Verification items for this drawing (mm, ordinates from the low corner). A direction names the side the tool comes from. Round coordinates to 2 decimals unless told otherwise and drop trailing zeros. Write each loop counter-clockwise with the first axis right and the second up, starting at its lowest first coordinate (ties: lowest second). Pieces come first, ordered by that corner, then holes. Notation, with made-up numbers: (-25, 48) -> (21, 48) arc R20 ccw to (21, 87) -> close; hole circle Ø5 at (60.5, 65). An arc over 180 degrees is marked (long way). Put each result on its own line as item: value. Start each with the question number.
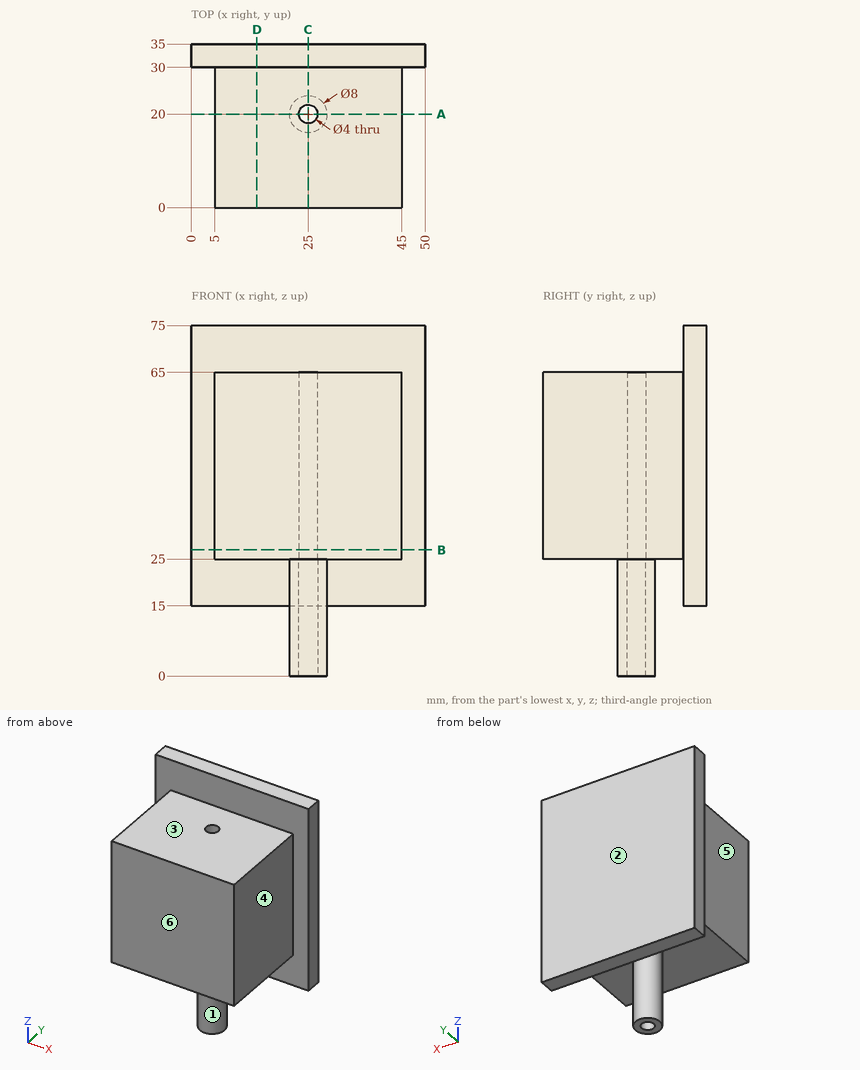
(1) Mould release check, pull along Y, two halves, no side actions. Record for the marked faces 1, 2 and 3: +Y half, -Y half, draft (parallel to the pull), parting line (faces both ways), or undercut.
(2) Sectioned sample at A-A (y = 20). Record the cut outline in (x, z).
(3) Go/stop test with flat-tipped pins: pin 1 Ø1.5 at (x, z) = (29, 10.5) entering from -Y; pin 2 Ø5.5 at (x, y) = (21, 32) entering from -Z; pin 3 Ø3 at (y, z) = (16, 16) entering from +X. Record where each tip stops, or that it passes through.
(4) Sectioned sample at D-D (x = 14). Record the cut outline in (y, z).
(5) Sectioned sample at C-C (x = 25). Record the cut outline in (y, z), and give its area (3 significant figures).
(6) Material ranges on L1, parallel to Y at x = 25, z = 52; L2, parallel to Y at x = 25, z = 6.5; L3, parallel to X at y = 20, z = 34, recorded low to high. Write a range as from..to.
(7) Set-up check for the marked faces 4, 5 and 6: record each of +Z, -Z, +X, -X, +Y, -Y from which the full face is reachable in a straight line by a thin tool's end or side.
(8) Sectioned sample at B-B (z = 27). Record the cut outline in (x, y).
Found:
1. face 1: undercut
1. face 2: +Y half
1. face 3: draft
2. outline: (5, 25) -> (21, 25) -> (21, 0) -> (23, 0) -> (23, 65) -> (5, 65) -> close; (27, 0) -> (29, 0) -> (29, 25) -> (45, 25) -> (45, 65) -> (27, 65) -> close
3. pin 1: y = 17.67
3. pin 2: z = 15
3. pin 3: x = 28.12
4. outline: (0, 25) -> (30, 25) -> (30, 15) -> (35, 15) -> (35, 75) -> (30, 75) -> (30, 65) -> (0, 65) -> close
5. outline: (0, 25) -> (16, 25) -> (16, 0) -> (18, 0) -> (18, 65) -> (0, 65) -> close; (22, 0) -> (24, 0) -> (24, 25) -> (30, 25) -> (30, 15) -> (35, 15) -> (35, 75) -> (30, 75) -> (30, 65) -> (22, 65) -> close
5. area: 1,440 mm2
6. L1: 0..18, 22..35
6. L2: 16..18, 22..24
6. L3: 5..23, 27..45
7. face 4: +Z, -Z, +X, -Y
7. face 5: +Z, -Z, -X, -Y
7. face 6: +Z, -Z, +X, -X, -Y
8. outline: (0, 30) -> (5, 30) -> (5, 0) -> (45, 0) -> (45, 30) -> (50, 30) -> (50, 35) -> (0, 35) -> close; hole circle Ø4 at (25, 20)
